For this review, take the finished solid that the model builds, in its own axes (mm). Face numbers are marked on the shaded views. A direction names the side the tool comes from. Round coordinates to 2 decimals unless told otherwise and drop trailing zeros. Write each loop counter-clockwise with the first axis right and the second up, starting at its lowest first coordinate (ties: lowest second). Pieces come first, ordered by that corner, then holes. Notation, with made-up numbers: (46.5, 55) -> (68.5, 55) arc R13 cw to (68.5, 70) -> close; hole circle Ø9 at (-11.75, 84.5). An arc over 180 degrees is marked (long way). Answer as CSV lines item,"result". Start each with the question number.
Item 1: Take a section at B-B on x = -36.5. Count the separate pieces of the cut face and the enclosed holes in it, then the cut area to 3 significant figures.
Item 2: Mouldability with a two-part tool opening along X and no side actions: class the marked faces 3, 4 and 5 as +X half, -X half, draft (parallel to the pull), parting line (faces both ways), or undercut.
Item 3: For pin 1 Ø2 at (x, y) = (15, -79) entering from +Z, flat-tipped, find the tip position at first contact; note if it passes through.
Item 4: Take a section at A-A on y = 115. Give the boundary of the cut face in (x, z), then the cut area to 4 significant figures.
Item 5: Wall thickness on probe 1 along Y at (x, z) = (44.5, 16.5); probe 2 along Z at (x, y) = (-69, 115); probe 3 along X at (y, z) = (77.5, 8.75): over which ranges is each line inside the solid? List them lowest first. Write a range as from..to.
Item 6: Machinability: for the marked faces 1 and 2, which of the approach directions +Z, -Z, +X, -X, +Y, -Y give a long, thin tool a straight path to every point of the face, cutting with its end or side? Answer none if there is none.
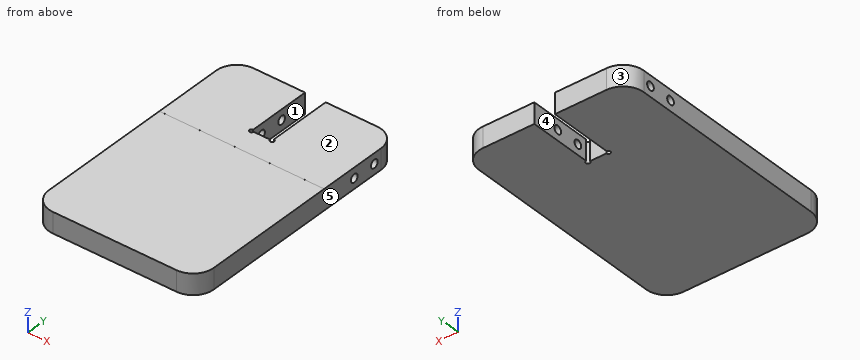
```python
from build123d import *

# Parameters (mm, degrees)
F1_DEPTH = 25
F2_R     = 5
F3_DEPTH = 200.001
F5_DEPTH = 0.01


with BuildPart() as f1:
    # F0 (on Top) → F1 (new body)
    with BuildSketch(Plane.XY):
        with BuildLine():
            Line((-12.5, 150), (-75, 150))
            ThreePointArc((-75, 150), (-92.67767, 142.67767), (-100, 125))
            Line((-100, 125), (-100, -125))
            ThreePointArc((-100, -125), (-92.67767, -142.67767), (-75, -150))
            Line((-75, -150), (75, -150))
            ThreePointArc((75, -150), (92.67767, -142.67767), (100, -125))
            Line((100, -125), (100, 125))
            ThreePointArc((100, 125), (92.67767, 142.67767), (75, 150))
            Line((75, 150), (12.5, 150))
            Line((12.5, 150), (12.5, 72.5))
            ThreePointArc((12.5, 72.5), (14.267767, 68.232233), (10, 70))
            Line((10, 70), (-10, 70))
            ThreePointArc((-10, 70), (-14.267767, 68.232233), (-12.5, 72.5))
            Line((-12.5, 72.5), (-12.5, 150))
        make_face()
    extrude(amount=F1_DEPTH)

    # F2 (on face) → F3 (cut, through all)
    with BuildSketch(Plane(origin=(-100, 0, 0), x_dir=(0, -1, 0), z_dir=(-1, 0, 0))):
        with Locations((-115, 12.5)):
            Circle(F2_R)
        with Locations((-85, 12.5)):
            Circle(F2_R)
    extrude(amount=-F3_DEPTH, mode=Mode.SUBTRACT)

    # F4 (on face) → F5 (cut)
    with BuildSketch(Plane.XY.offset(25)):
        with BuildLine():
            ThreePointArc((-100, -125), (-92.67767, -142.67767), (-75, -150))
            Line((-75, -150), (75, -150))
            ThreePointArc((75, -150), (92.67767, -142.67767), (100, -125))
            Line((100, -125), (100, 40))
            Line((100, 40), (-100, 40))
            Line((-100, 40), (-100, -125))
        make_face()
    extrude(amount=-F5_DEPTH, mode=Mode.SUBTRACT)


solid = f1.part
```
Output values:
1,separate pieces,"1"
1,enclosed holes,"2"
1,area,"7,340 mm^2"
2,face 3,"-X half"
2,face 4,"undercut"
2,face 5,"+X half"
3,pin 1,"stops at z = 24.99"
4,outline,"(-100, 0) -> (-12.5, 0) -> (-12.5, 7.5) -> (-100, 7.5) -> close; (-100, 17.5) -> (-12.5, 17.5) -> (-12.5, 25) -> (-100, 25) -> close; (12.5, 0) -> (100, 0) -> (100, 7.5) -> (12.5, 7.5) -> close; (12.5, 17.5) -> (100, 17.5) -> (100, 25) -> (12.5, 25) -> close"
4,area,"2,625 mm^2"
5,probe 1,"y = -150..82, 88..112, 118..150"
5,probe 2,"z = 0..7.5, 17.5..25"
5,probe 3,"x = -100..-12.5, 12.5..100"
6,face 1,"+Z, -Z, +Y"
6,face 2,"+Z, +X, -X, +Y, -Y"
